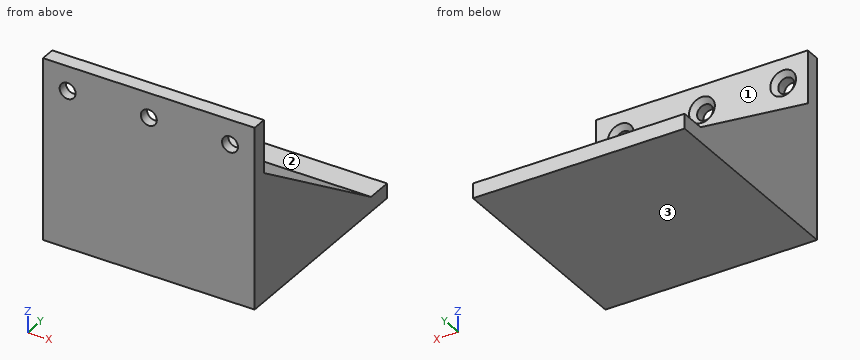
```python
from build123d import *

# Parameters (mm, degrees)
SCHIZZO1_W                   = 43
SCHIZZO1_H                   = 43
ESTRUSIONE_ESTRUSIONE1_DEPTH = 3
ESTRUSIONE_ESTRUSIONE2_DEPTH = 43
SCHIZZO3_R                   = 1.62
TAGLIO_ESTRUSIONE1_DEPTH     = 43
SMUSSO1_SIZE                 = 1
SCHIZZO3_3_R                 = 1.62
TAGLIO_ESTRUSIONE2_DEPTH     = 43
SCHIZZO3_4_R                 = 1.62
TAGLIO_ESTRUSIONE3_DEPTH     = 43
SMUSSO2_SIZE                 = 1
SMUSSO3_SIZE                 = 1


with BuildPart() as part:
    # Schizzo1 → Estrusione-Estrusione1 (new body)
    with BuildSketch(Plane.XY):
        Rectangle(SCHIZZO1_W, SCHIZZO1_H)
    extrude(amount=ESTRUSIONE_ESTRUSIONE1_DEPTH)

    # Schizzo2 → Estrusione-Estrusione2 (add)
    with BuildSketch(Plane.ZY.offset(21.5)):
        Polygon((26.100411225, -18.5), (3, 16.313408291), (3, -21.5), (36.837031378, -21.5), (36.837031378, -18.5), align=None)
    extrude(amount=-ESTRUSIONE_ESTRUSIONE2_DEPTH)

    # Schizzo3 → Taglio-Estrusione1 (cut)
    with BuildSketch(Plane(origin=(0, -18.5, 0), x_dir=(1, 0, 0), z_dir=(0, 1, 0))):
        with Locations(Location((16.5, -31.837031378, 0), (0, 0, 180))):
            Circle(SCHIZZO3_R)
    extrude(amount=-TAGLIO_ESTRUSIONE1_DEPTH, mode=Mode.SUBTRACT)

    # Smusso1
    smusso1_edges = [part.edges().sort_by_distance(p)[0] for p in [
        (18.12, -18.5, 31.837031378),
    ]]
    chamfer(smusso1_edges, length=SMUSSO1_SIZE)

    # Schizzo3_3 → Taglio-Estrusione2 (cut)
    with BuildSketch(Plane(origin=(0, -18.5, 0), x_dir=(1, 0, 0), z_dir=(0, 1, 0))):
        with Locations(Location((0, -31.837031378, 0), (0, 0, 180))):
            Circle(SCHIZZO3_3_R)
    extrude(amount=-TAGLIO_ESTRUSIONE2_DEPTH, mode=Mode.SUBTRACT)

    # Schizzo3_4 → Taglio-Estrusione3 (cut)
    with BuildSketch(Plane(origin=(0, -18.5, 0), x_dir=(1, 0, 0), z_dir=(0, 1, 0))):
        with Locations(Location((-16.5, -31.837031378, 0), (0, 0, 180))):
            Circle(SCHIZZO3_4_R)
    extrude(amount=-TAGLIO_ESTRUSIONE3_DEPTH, mode=Mode.SUBTRACT)

    # Smusso2
    smusso2_edges = [part.edges().sort_by_distance(p)[0] for p in [
        (1.62, -18.5, 31.837031378),
    ]]
    chamfer(smusso2_edges, length=SMUSSO2_SIZE)

    # Smusso3
    smusso3_edges = [part.edges().sort_by_distance(p)[0] for p in [
        (-14.88, -18.5, 31.837031378),
    ]]
    chamfer(smusso3_edges, length=SMUSSO3_SIZE)


solid = part.part
```
The listing builds one solid part. Answer for the finished solid, in the listing's coordinates (mm). Face numbers are marked on the shaded views. Coordinates: 2 decimals unless noted, no trailing zeros. Write each loop counter-clockwise with the first axis right and the second up, starting at its lowest first coordinate (ties: lowest second). Pieces come first, ordered by that corner, then holes.
Q1. Find the intervals of material crossed by line 1 along Z through (x, y) = (-16.5, -20.45); line 2 along Z through (x, y) = (5.5, 18); line 3 along Z through (x, y) = (16, -20), in increasing order.
Returned:
line 1: z = 0 to 30.22, 33.46 to 36.84
line 2: z = 0 to 3
line 3: z = 0 to 30.3, 33.38 to 36.84
Q2. Section D-D, the plane z = 17.5 is taken. Write down the section's boundary in (x, y), then the cut area to 3 significant figures.
Returned:
outline: (-21.5, -21.5) - (21.5, -21.5) - (21.5, -5.54) - (-21.5, -5.54) - close
area: 686 mm2
Q3. Section C-C, the plane y = -0.5 is taken. Write down the section's boundary in (x, z).
Returned:
outline: (-21.5, 0) - (21.5, 0) - (21.5, 14.16) - (-21.5, 14.16) - close
Q4. Given P1, Ø8, axis at x = 16, z = 7.5, coming from the +Y side; P2, Ø12, axis at x = -4, z = 29, coming from the +Y side; P3, Ø2.5, axis at x = 6.5, y = 20, coming from the +Z side, each flat-ended and moving along its own axis, determine where each tip first touches the part or whether it passes through.
Returned:
P1: stops at y = 15.56
P2: stops at y = -13.83
P3: stops at z = 3
Q5. The mould has two halves that part along Z. Classify the marked faces 1, 2 and 3: released by +Z, released by -Z, zero draft, split by the parting line, or undercut.
Returned:
face 1: zero draft
face 2: released by +Z
face 3: released by -Z
Q6. Section A-A, the plane x = 16.5 is taken. Write down the section's boundary in (y, z), then the cut area to 3 significant figures.
Returned:
outline: (-21.5, 0) - (21.5, 0) - (21.5, 3) - (16.31, 3) - (-18.5, 26.1) - (-18.5, 29.22) - (-19.5, 30.22) - (-21.5, 30.22) - close; (-21.5, 33.46) - (-19.5, 33.46) - (-18.5, 34.46) - (-18.5, 36.84) - (-21.5, 36.84) - close
area: 622 mm2
Q7. Section B-B, the plane x = 10 is taken. Write down the section's boundary in (y, z).
Returned:
outline: (-21.5, 0) - (21.5, 0) - (21.5, 3) - (16.31, 3) - (-18.5, 26.1) - (-18.5, 36.84) - (-21.5, 36.84) - close
